Build history of the part. All positions in model axes, mm. Face numbers are marked on the shaded views. A direction names the side the tool comes from. Give positions to 0.01 mm unless a question says otherwise; leave off trailing zeros. Loops run counter-clockwise (first coordinate to the right, second up) from the corner with the lowest first, then second, coordinate; pieces in that order, holes last. Notation, with made-up numbers: M -13,-20.5 L 28,-20.5 A8 ccw 28,-8.5 Z; hole C 2,33.25 d1. An arc over 180 degrees is marked long. Answer as a JSON object with one key per item and string values. Group by question number.
1. Drill centre lines: line 1 along Y through (x, z) = (5.5, -3); line 2 along Y through (x, z) = (-3.25, 4.5); line 3 along Z through (x, y) = (0.25, 23.5). Where is each one in solid material? Low to high. Write a range as [from, to].
2. Slice it at B-B (y = 4). List the corners of the cut face in (x, z).
3. 3-axis set-ups, long thin cutter, end or side, ignore diameter. For the marked faces 1, 2 and 3: which of +Z, -Z, +X, -X, +Y, -Y reach the whole face in a straight line?
4. Slice it at A-A (x = 0). List the corners of the cut face in (y, z), then the cut area to 3 significant figures.
5. Drop flat-ended pins along their axis: pin 1 Ø1 at (x, z) = (6.5, -2) entering from -Y; pin 2 Ø6 at (y, z) = (6, -1) entering from -X; pin 3 Ø1 at (y, z) = (25.5, 1.5) entering from +X. Give the stop position or say it passes through.
6. Slice it at C-C (y = 27.5). List the corners of the cut face in (x, z), then the cut area to 3 significant figures.
from build123d import *

# Parameters (mm, degrees)
SKETCH1_R           = 5.85
BOSS_EXTRUDE1_DEPTH = 17.2
SKETCH2_R           = 9
BOSS_EXTRUDE2_DEPTH = 2.5
BOSS_EXTRUDE2_TAPER = 56
SKETCH3_R           = 5
BOSS_EXTRUDE3_DEPTH = 3.5
SKETCH4_R           = 6.9
BOSS_EXTRUDE4_DEPTH = 7.5
SKETCH5_OUTSIDE_W   = 27.976
SKETCH5_OUTSIDE_H   = 27.976
SKETCH5_OUTSIDE_R   = 5.15
CUT_EXTRUDE1_DEPTH  = 11.2


with BuildPart() as part:
    # Sketch1 → Boss-Extrude1 (new body)
    with BuildSketch(Plane(origin=(0, 0, 0), x_dir=(1, 0, 0), z_dir=(0, 1, 0))):
        with Locations(Location((0, 0, 0), (0, 0, 270))):  # turned: the seam where the file's is
            Circle(SKETCH1_R)
    extrude(amount=BOSS_EXTRUDE1_DEPTH)

    # Sketch2 → Boss-Extrude2 (add)
    with BuildSketch(Plane(origin=(0, 17.2, 0), x_dir=(1, 0, 0), z_dir=(0, 1, 0))):
        Circle(SKETCH2_R)
    extrude(amount=BOSS_EXTRUDE2_DEPTH, taper=BOSS_EXTRUDE2_TAPER)

    # Sketch3 → Boss-Extrude3 (add)
    with BuildSketch(Plane(origin=(0, 19.7, 0), x_dir=(1, 0, 0), z_dir=(0, 1, 0))):
        with Locations(Location((0, 0, 0), (0, 0, 270))):  # turned: the seam where the file's is
            Circle(SKETCH3_R)
    extrude(amount=BOSS_EXTRUDE3_DEPTH)

    # Sketch4 → Boss-Extrude4 (add)
    with BuildSketch(Plane(origin=(0, 23.2, 0), x_dir=(1, 0, 0), z_dir=(0, 1, 0))):
        with Locations(Location((0, 0, 0), (0, 0, 270))):  # turned: the seam where the file's is
            Circle(SKETCH4_R)
    extrude(amount=BOSS_EXTRUDE4_DEPTH)

    # Sketch5 outside → Cut-Extrude1 (cut)
    with BuildSketch(Plane.XZ):
        Rectangle(SKETCH5_OUTSIDE_W, SKETCH5_OUTSIDE_H)
        with Locations(Location((0, 0, 0), (0, 0, 270))):  # turned: the seam where the file's is
            Circle(SKETCH5_OUTSIDE_R, mode=Mode.SUBTRACT)
    extrude(amount=-CUT_EXTRUDE1_DEPTH, mode=Mode.SUBTRACT)


solid = part.part
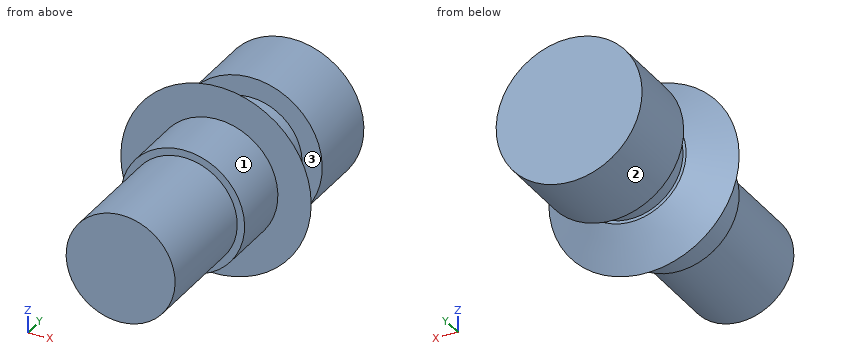
Established:
{
 "1": {"line 1": "y = [17.2, 19.04], [23.2, 30.7]", "line 2": "y = [11.2, 19.53], [23.2, 30.7]", "line 3": "z = [-6.9, 6.9]"},
 "2": {"outline": "C 0,0 d10.3"},
 "3": {"face 1": "-Y", "face 2": "+Y", "face 3": "none"},
 "4": {"outline": "M 0,-5.15 L 11.2,-5.15 L 11.2,-5.85 L 17.2,-5.85 L 17.2,-9 L 19.7,-5.29 L 19.7,-5 L 23.2,-5 L 23.2,-6.9 L 30.7,-6.9 L 30.7,6.9 L 23.2,6.9 L 23.2,5 L 19.7,5 L 19.7,5.29 L 17.2,9 L 17.2,5.85 L 11.2,5.85 L 11.2,5.15 L 0,5.15 Z", "area": "360 mm^2"},
 "5": {"pin 1": "stops at y = 17.2", "pin 2": "stops at x = -5.15", "pin 3": "stops at x = 6.83"},
 "6": {"outline": "C 0,0 d13.8", "area": "150 mm^2"}
}
